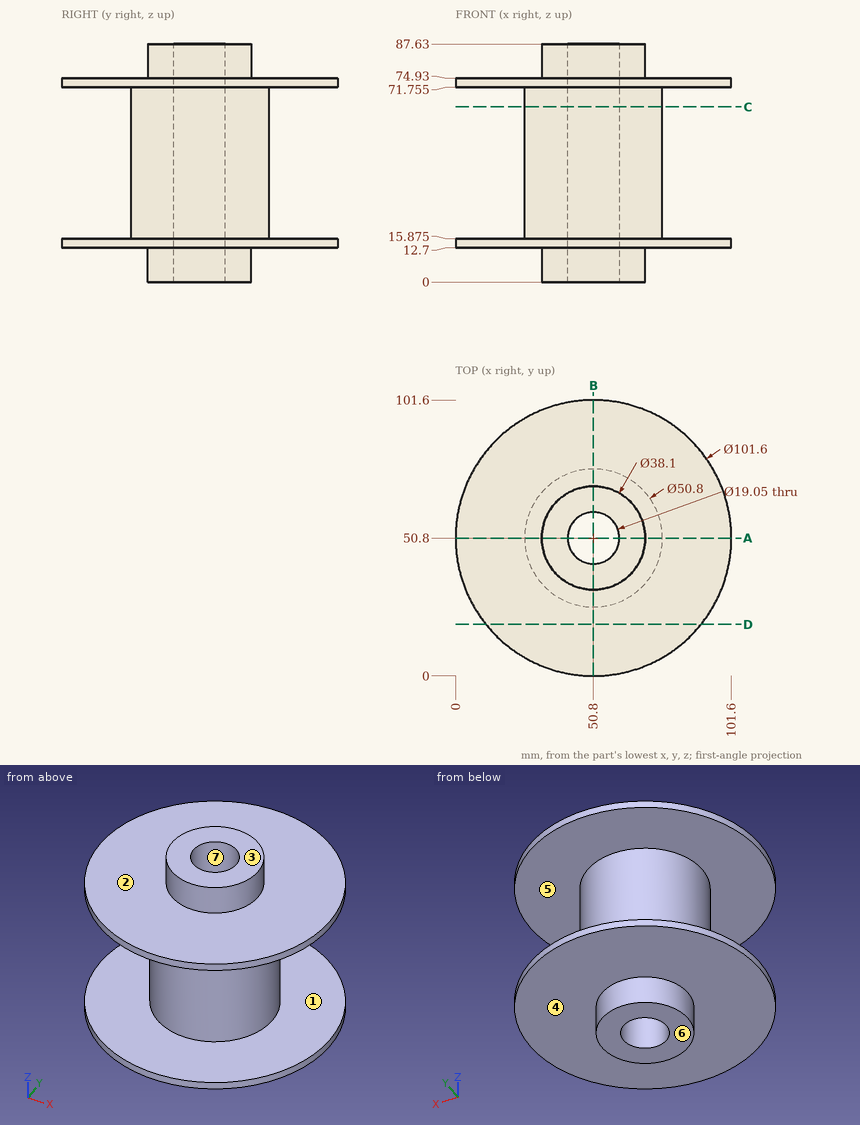
Print and shaded views of the part. All mm, measured from the part's lowest x, y and z. A direction names the side the tool comes from. Give positions to 0.01 mm unless a question says otherwise; leave off trailing zeros. Order: outer loops, then holes, each group sorted by start corner. A loop starts at its lowest first (then second) coordinate and runs counter-clockwise, first axis right, second up. Notation, with made-up numbers: (6.25, 27) - (47.25, 27) arc R15 ccw to (47.25, 34) - close; hole circle Ø11 at (-27.5, 13). An arc over 180 degrees is marked (long way). Use a Markdown table: item, result.
1) Saw through at D-D on y = 19. List the corners of the cut face in (x, z) (3 decimals), plus the area to 3 significant figures.
Checked values:
| item | result |
|---|---|
| outline | (11.184, 12.7) - (90.416, 12.7) - (90.416, 15.875) - (11.184, 15.875) - close; (11.184, 71.755) - (90.416, 71.755) - (90.416, 74.93) - (11.184, 74.93) - close |
| area | 503 mm² |
2) 3-axis set-ups, long thin cutter, end or side, ignore diameter. For the marked faces 1, 2, 3 and 4: which of +Z, -Z, +X, -X, +Y, -Y reach the whole face in a straight line?
Checked values:
| item | result |
|---|---|
| face 1 | none |
| face 2 | +Z |
| face 3 | +Z, +X, -X, +Y, -Y |
| face 4 | -Z |
3) Saw through at A-A on y = 50.8. List the corners of the cut face in (x, z) (3 decimals), plus the area to 3 significant figures.
Checked values:
| item | result |
|---|---|
| outline | (0, 12.7) - (31.75, 12.7) - (31.75, 0) - (41.275, 0) - (41.275, 87.63) - (31.75, 87.63) - (31.75, 74.93) - (0, 74.93) - (0, 71.755) - (25.4, 71.755) - (25.4, 15.875) - (0, 15.875) - close; (60.325, 0) - (69.85, 0) - (69.85, 12.7) - (101.6, 12.7) - (101.6, 15.875) - (76.2, 15.875) - (76.2, 71.755) - (101.6, 71.755) - (101.6, 74.93) - (69.85, 74.93) - (69.85, 87.63) - (60.325, 87.63) - close |
| area | 2,780 mm² |
4) Probe L1, parallel to Y at x = 50.8, z = 54 (3 decimals); L2, parallel to Z at x = 55, y = 24 (3 decimals); L3, parallel to X at y = 50, z = 61. List the from-to ranges inside material, lowest first. Write a range as from..to.
Checked values:
| item | result |
|---|---|
| L1 | 25.4..41.275, 60.325..76.2 |
| L2 | 12.7..15.875, 71.755..74.93 |
| L3 | 25.41..41.31, 60.29..76.19 |
5) Two-plate mould, pull along Z, no slides. Class the marked faces 5, 6 and 7: +Z half, -Z half, draft (parallel to the pull), parting line (faces both ways), or undercut.
Checked values:
| item | result |
|---|---|
| face 5 | undercut |
| face 6 | -Z half |
| face 7 | draft |
6) Flat gauge pins, fed straight in: P1, Ø3, axis at x = 73.5, y = 60.5, coming from the -Z side; P2, Ø4, axis at y = 79.5, z = 70, coming from the -X side; P3, Ø3, axis at y = 53, z = 75.5, coming from the +X side. Where does each tip first touch, or does it go through?
Checked values:
| item | result |
|---|---|
| P1 | z = 12.7 |
| P2 | x = 8.24 |
| P3 | x = 101.59 |
7) Saw through at C-C on z = 64.5. List the corners of the cut face in (x, y) (3 decimals), plus the area to 3 significant figures.
Checked values:
| item | result |
|---|---|
| outline | circle Ø50.8 at (50.8, 50.8); hole circle Ø19.05 at (50.8, 50.8) |
| area | 1,740 mm² |
